from build123d import *

# Parameters (mm, degrees)
SKETCH1_W           = 328.60742
SKETCH1_H           = 111.6203
SKETCH1_W_2         = 271.033754468
SKETCH1_H_2         = 2.54
SKETCH1_W_3         = 2.54
SKETCH1_H_3         = 70.9803
BOSS_EXTRUDE1_DEPTH = 2.286
SKETCH2_W           = 328.60742
SKETCH2_H           = 50.8
BOSS_EXTRUDE2_DEPTH = 2.286


with BuildPart() as part:
    # Sketch1 → Boss-Extrude1 (new body)
    with BuildSketch(Plane.XY):
        with Locations((156.68371, 48.19015)):
            Rectangle(SKETCH1_W, SKETCH1_H)
        with Locations((156.68371, 97.6503)):
            Rectangle(SKETCH1_W_2, SKETCH1_H_2, mode=Mode.SUBTRACT)
        with Locations((-1.27, 48.19015)):
            Rectangle(SKETCH1_W_3, SKETCH1_H_3, mode=Mode.SUBTRACT)
        with Locations((314.63742, 48.19015)):
            Rectangle(SKETCH1_W_3, SKETCH1_H_3, mode=Mode.SUBTRACT)
        with Locations((156.68371, -1.27)):
            Rectangle(SKETCH1_W_2, SKETCH1_H_2, mode=Mode.SUBTRACT)
    extrude(amount=BOSS_EXTRUDE1_DEPTH)

    # Sketch2 → Boss-Extrude2 (add, through all)
    with BuildSketch(Plane.XY.offset(2.286)):
        with Locations((156.68371, 129.4003)):
            Rectangle(SKETCH2_W, SKETCH2_H)
        with Locations((156.68371, -33.02)):
            Rectangle(SKETCH2_W, SKETCH2_H)
    extrude(amount=-BOSS_EXTRUDE2_DEPTH)


solid = part.part
The model under review builds one solid part; all positions refer to its coordinate system, in mm. Round coordinates to 2 decimals unless told otherwise and drop trailing zeros. Loops run counter-clockwise (first coordinate to the right, second up) from the corner with the lowest first, then second, coordinate; pieces in that order, holes last. Notation, with made-up numbers: (36, 14.5) - (48, 14.5) arc R13 cw to (48, 33.5) - close; hole circle Ø4 at (-25.5, 24.5). An arc over 180 degrees is marked (long way). Use CSV: the item, a comma, the result in double quotes.
(1) Take a section at A-A, the plane x = 201. Give the boundary of the cut face in (y, z), plus the area to 3 significant figures.
Working result:
outline,"(-58.42, 0) - (-2.54, 0) - (-2.54, 2.29) - (-58.42, 2.29) - close; (0, 0) - (96.38, 0) - (96.38, 2.29) - (0, 2.29) - close; (98.92, 0) - (154.8, 0) - (154.8, 2.29) - (98.92, 2.29) - close"
area,"476 mm^2"
(2) Take a section at C-C, the plane y = 80.5. Give the boundary of the cut face in (x, z), plus the area to 3 significant figures.
Working result:
outline,"(-7.62, 0) - (-2.54, 0) - (-2.54, 2.29) - (-7.62, 2.29) - close; (0, 0) - (313.37, 0) - (313.37, 2.29) - (0, 2.29) - close; (315.91, 0) - (320.99, 0) - (320.99, 2.29) - (315.91, 2.29) - close"
area,"740 mm^2"
(3) For line 1 (Y direction, x = 215, z = 0.5); line 2 (X direction, y = 43, z = 1); line 3 (X direction, y = 97.5, z = 0.35), list the stretches that pass through material, from the lowest coordinate up.
Working result:
line 1,"y = -58.42 to -2.54, 0 to 96.38, 98.92 to 154.8"
line 2,"x = -7.62 to -2.54, 0 to 313.37, 315.91 to 320.99"
line 3,"x = -7.62 to 21.17, 292.2 to 320.99"
(4) Take a section at B-B, the plane z = 0.7. Give the boundary of the cut face in (x, y), plus the area to 3 significant figures.
Working result:
outline,"(-7.62, -58.42) - (320.99, -58.42) - (320.99, 154.8) - (-7.62, 154.8) - close; hole (-2.54, 12.7) - (0, 12.7) - (0, 83.68) - (-2.54, 83.68) - close; hole (21.17, -2.54) - (292.2, -2.54) - (292.2, 0) - (21.17, 0) - close; hole (21.17, 96.38) - (292.2, 96.38) - (292.2, 98.92) - (21.17, 98.92) - close; hole (313.37, 12.7) - (315.91, 12.7) - (315.91, 83.68) - (313.37, 83.68) - close"
area,"68,300 mm^2"
